```python
from build123d import *

# Parameters (mm, degrees)
F1_DEPTH = 63.5
F0_W     = 2.669878304
F0_H     = 19.05
F2_DEPTH = 25.4
F3_DEPTH = 7.9375
F5_R     = 5.08


# Not quite as in the source:
# - a feature of the source that left no trace in its solid (it failed there, or was rolled back) is left out


with BuildPart() as f1:
    # F0 (on Front) → F1 (new body, symmetric)
    with BuildSketch(Plane.XZ):
        Polygon((22.225, 9.525), (-41.275, 9.525), (-41.275, -9.525), (41.275, -9.525), (41.275, 9.525), align=None)
    extrude(amount=F1_DEPTH, both=True)

    # F0 (on Front) → F2 (join, symmetric)
    with BuildSketch(Plane.XZ):
        with BuildLine():
            Line((22.225, 34.3503219656), (22.225, 9.525))
            Line((22.225, 9.525), (41.275, 9.525))
            Line((41.275, 9.525), (41.275, 34.3503219656))
            ThreePointArc((41.275, 34.3503219656), (45.9246798487, 45.5756421169), (57.15, 50.2253219656))
            Line((57.15, 50.2253219656), (71.9948219351, 50.2253219656))
            Line((71.9948219351, 50.2253219656), (71.9948219351, 69.2753219656))
            Line((71.9948219351, 69.2753219656), (57.15, 69.2753219656))
            ThreePointArc((57.15, 69.2753219656), (32.4542956671, 59.0460262985), (22.225, 34.3503219656))
        make_face()
        with Locations((73.3297610871, 59.7503219656)):
            Rectangle(F0_W, F0_H)
    extrude(amount=F2_DEPTH, both=True)

    # F0 (on Front) → F3 (join, symmetric)
    with BuildSketch(Plane.XZ):
        with BuildLine():
            add(Edge.make_bspline(
                [(-41.275, 9.525), (8.1134410575, 11.8744410574), (14.8591641337, 70.7333981991), (57.15, 69.2753219656)],
                knots=[0, 0, 0, 0, 115.1415719885, 115.1415719885, 115.1415719885, 115.1415719885], degree=3))
            Line((-41.275, 9.525), (22.225, 9.525))
            Line((22.225, 9.525), (22.225, 34.3503219656))
            ThreePointArc((22.225, 34.3503219656), (32.4542956671, 59.0460262985), (57.15, 69.2753219656))
        make_face()
    extrude(amount=F3_DEPTH, both=True)

    # F5
    f5_edges = [f1.edges().sort_by_distance(p)[0] for p in [
        (-41.275, -63.5, 0),
        (-41.275, 63.5, 0),
        (41.275, -63.5, 0),
        (41.275, 63.5, 0),
    ]]
    fillet(f5_edges, radius=F5_R)


solid = f1.part
```
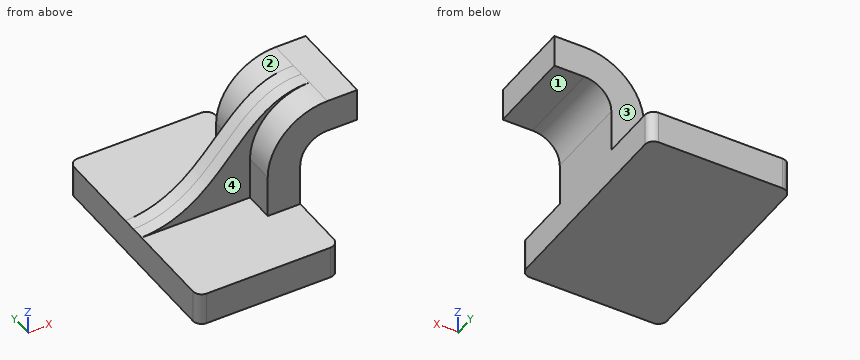
CAD build for the part. Positions are in the model's coordinates, mm. Face numbers are marked on the shaded views. A direction names the side the tool comes from. Give positions to 0.01 mm unless a question says otherwise; leave off trailing zeros. Order: outer loops, then holes, each group sorted by start corner. A loop starts at its lowest first (then second) coordinate and runs counter-clockwise, first axis right, second up. Notation, with made-up numbers: M 29,-13.5 L 76,-13.5 A35 cw 76,19.5 Z; hole C 49.25,-40 d2. An arc over 180 degrees is marked long. Put each result on its own line as item: value. Start each with the question number.
(1) Saw through at A-A, the plane z = 7.5. Write the cut outline in (x, y) (3 decimals).
(2) Saw through at D-D, the plane y = 45. Write the cut outline in (x, z) (3 decimals).
(3) Drill centre lines: line 1 along Z through (x, y) = (29.5, -35.5) (3 decimals); line 2 along Y through (x, z) = (41, 51); line 3 along Y through (x, z) = (9, 35). Where is each one in solid material? Low to high.
(4) Which spindle directions (+Z, -Z, +X, -X, +Y, -Y) get a long thin tool onto all of the face, cutting with end or side? Do the marked faces 1, 2, 3 and 4. Say none if no direction does.
(5) Saw through at C-C, the plane x = 63.5. Write the cut outline in (y, z).
(6) Saw through at B-B, the plane y = -12.5. Write the cut outline in (x, z) (3 decimals), then the cut area to 3 significant figures.
(7) Flat gauge pins, fed straight in: pin 1 Ø9 at (x, y) = (63.5, 1) entering from +Z; pin 2 Ø15.5 at (x, z) = (52.5, 49.5) entering from -Y; pin 3 Ø1 at (y, z) = (9, 21.5) entering from +X (3 decimals). Where does each tip first touch, or does it go through?
Check result:
1. outline: M -41.275,-58.42 A5.08 ccw -36.195,-63.5 L 36.195,-63.5 A5.08 ccw 41.275,-58.42 L 41.275,58.42 A5.08 ccw 36.195,63.5 L -36.195,63.5 A5.08 ccw -41.275,58.42 Z
2. outline: M -41.275,-9.525 L 41.275,-9.525 L 41.275,9.525 L -41.275,9.525 Z
3. line 1: z = -9.525 to 9.525
3. line 2: y = -25.4 to 25.4
3. line 3: y = -7.94 to 7.94
4. face 1: -Z, +X, +Y, -Y
4. face 2: +Z, -X, +Y
4. face 3: +Z, +X, -X, +Y
4. face 4: +Z, -X, -Y
5. outline: M -25.4,50.23 L 25.4,50.23 L 25.4,69.28 L -25.4,69.28 Z
6. outline: M -41.275,-9.525 L 41.275,-9.525 L 41.275,34.35 A15.875 cw 57.15,50.225 L 74.665,50.225 L 74.665,69.275 L 57.15,69.275 A34.925 ccw 22.225,34.35 L 22.225,9.525 L -41.275,9.525 Z
6. area: 3,140 mm2
7. pin 1: stops at z = 69.28
7. pin 2: stops at y = -25.4
7. pin 3: stops at x = 41.275
